from build123d import *

# Parameters (mm, degrees)
SKETCH1_W           = 203
SKETCH1_H           = 90
BOSS_EXTRUDE1_DEPTH = 5
SKETCH3_W           = 5
SKETCH3_H           = 25
SKETCH3_W_2         = 101
SKETCH3_H_2         = 5
CUT_EXTRUDE2_DEPTH  = 223.112584065
SKETCH4_W           = 193
SKETCH4_H           = 3
CUT_EXTRUDE3_DEPTH  = 2.5
SKETCH5_W           = 3.1
SKETCH5_H           = 1.8
SKETCH5_W_2         = 1.15
SKETCH5_H_2         = 2.2
SKETCH5_H_3         = 2
CUT_EXTRUDE4_DEPTH  = 223.112584065


with BuildPart() as part:
    # Sketch1 → Boss-Extrude1 (new body)
    with BuildSketch(Plane.XY):
        with Locations((101.5, 45)):
            Rectangle(SKETCH1_W, SKETCH1_H)
    extrude(amount=BOSS_EXTRUDE1_DEPTH)

    # Sketch3 → Cut-Extrude2 (cut, through all)
    with BuildSketch(Plane(origin=(0, 0, 0), x_dir=(-1, 0, 0), z_dir=(0, 0, -1))):
        with Locations((-200.5, 12.5)):
            Rectangle(SKETCH3_W, SKETCH3_H)
        with Locations((-200.5, 77.5)):
            Rectangle(SKETCH3_W, SKETCH3_H)
        with Locations((-2.5, 12.5)):
            Rectangle(SKETCH3_W, SKETCH3_H)
        with Locations((-2.5, 77.5)):
            Rectangle(SKETCH3_W, SKETCH3_H)
        with Locations((-101.5, 2.5)):
            Rectangle(SKETCH3_W_2, SKETCH3_H_2)
    extrude(amount=-CUT_EXTRUDE2_DEPTH, mode=Mode.SUBTRACT)

    # Sketch4 → Cut-Extrude3 (cut)
    with BuildSketch(Plane(origin=(0, 0, 0), x_dir=(-1, 0, 0), z_dir=(0, 0, -1))):
        with Locations((-101.5, 86)):
            Rectangle(SKETCH4_W, SKETCH4_H)
    extrude(amount=-CUT_EXTRUDE3_DEPTH, mode=Mode.SUBTRACT)

    # Sketch5 → Cut-Extrude4 (cut, through all)
    with BuildSketch(Plane(origin=(0, 0, 0), x_dir=(-1, 0, 0), z_dir=(0, 0, -1))):
        with Locations((-101.5, 10.1)):
            Rectangle(SKETCH5_W, SKETCH5_H)
        with Locations((-103.625, 8.1)):
            Rectangle(SKETCH5_W_2, SKETCH5_H_2)
        with Locations((-101.5, 8.1)):
            Rectangle(SKETCH5_W, SKETCH5_H_2)
        with Locations((-99.375, 8.1)):
            Rectangle(SKETCH5_W_2, SKETCH5_H_2)
        with Locations((-101.5, 6)):
            Rectangle(SKETCH5_W, SKETCH5_H_3)
    extrude(amount=-CUT_EXTRUDE4_DEPTH, mode=Mode.SUBTRACT)


solid = part.part
Input: part model. Units: mm. Frame: model coordinates. A direction names the side the tool comes from. Coordinates: 2 decimals unless noted, no trailing zeros. Loops run counter-clockwise (first coordinate to the right, second up) from the corner with the lowest first, then second, coordinate; pieces in that order, holes last.
(1) Section B-B on x = 144. Return the cut outline in (y, z).
(2) Set-up query: faces 1 (the face through (5, 77, 2)), 2 (the face through (152, 2, 2)), 3 (the face through (3, 25, 2)), 4 (the face through (198, 12, 2)), 5 (the face through (198, 77, 2)). Return all of +Z, -Z, +X, -X, +Y, -Y with unobstructed straight access to the full face (end or side cutting, diameter ignored); none if empty.
(3) Section C-C on x = 178. Return the cut outline in (y, z).
(4) First-contact query: pin 1 Ø8 at (x, y) = (57, 76.5) entering from -Z; pin 2 Ø1.6 at (y, z) = (6, 3) entering from -X; pin 3 Ø2 at (x, z) = (68.5, 4) entering from -Y; pin 4 Ø1.6 at (y, z) = (6.5, 2.5) entering from +X. Flat tips, straight axial feed; report the tip coordinate or a pass-through.
(5) Material intervals for probe 1 along Y at (x, z) = (33.5, 0.85); probe 2 along Y at (x, z) = (134.5, 0.4); probe 3 along Y at (x, z) = (102.5, 4.65), sorted ascending.
(6) Section D-D on y = 71. Return the cut outline in (x, z), then the cut area to 3 significant figures.
Data:
1. outline: (5, 0) - (84.5, 0) - (84.5, 2.5) - (87.5, 2.5) - (87.5, 0) - (90, 0) - (90, 5) - (5, 5) - close
2. face 1: +Z, -Z, -X, +Y
2. face 2: +Z, -Z, -Y
2. face 3: +Z, -Z, -X, -Y
2. face 4: +Z, -Z, +X, -Y
2. face 5: +Z, -Z, +X, +Y
3. outline: (0, 0) - (84.5, 0) - (84.5, 2.5) - (87.5, 2.5) - (87.5, 0) - (90, 0) - (90, 5) - (0, 5) - close
4. pin 1: stops at z = 0
4. pin 2: stops at x = 5
4. pin 3: stops at y = 5
4. pin 4: stops at x = 198
5. probe 1: y = 0 to 84.5, 87.5 to 90
5. probe 2: y = 5 to 84.5, 87.5 to 90
5. probe 3: y = 11 to 90
6. outline: (5, 0) - (198, 0) - (198, 5) - (5, 5) - close
6. area: 965 mm2
